Source: CAD feature listing. Evaluate the final solid. Frame: model axes, mm. A direction names the side the tool comes from. Round coordinates to 2 decimals unless told otherwise and drop trailing zeros. Loops run counter-clockwise (first coordinate to the right, second up) from the corner with the lowest first, then second, coordinate; pieces in that order, holes last. Notation, with made-up numbers: M 78.25,-39.5 L 110.25,-39.5 A22 cw 110.25,-12.5 Z; hole C 15.5,-28 d3. An arc over 180 degrees is marked long. One line per item, written item: value.
from build123d import *

# Parameters (mm, degrees)
F0_R     = 2
F1_DEPTH = 25
F2_R     = 12.5
F2_R_2   = 2
F3_DEPTH = 7.5


with BuildPart() as f1:
    # F0 (on Top) → F1 (new body)
    with BuildSketch(Plane.XY):
        Circle(F0_R)
    extrude(amount=F1_DEPTH)

    # F2 (on face) → F3 (join, symmetric)
    with BuildSketch(Plane.XY.offset(25)):
        Circle(F2_R)
        Circle(F2_R_2, mode=Mode.SUBTRACT)
    extrude(amount=F3_DEPTH, both=True)


solid = f1.part
1. Pull-direction query (Y, two-part tool) for faces 3 (the face through (0, -3, 17.5)), 4 (the face through (0, -2, 9)), 5 (the face through (0, 0, 25)); classes: released by +Y, released by -Y, zero draft, split by the parting line, or undercut.
Report:
face 3: zero draft
face 4: split by the parting line
face 5: undercut
2. Ray query, line 1 (Y direction, x = 0, z = 27); line 2 (Z direction, x = 7.5, y = -0.25); line 3 (Z direction, x = 0.75, y = -1.25). Return the intervals inside material, ascending. Write a range as [from, to].
Report:
line 1: y = [-12.5, -2], [2, 12.5]
line 2: z = [17.5, 32.5]
line 3: z = [0, 25]
3. Section query C-C (z = 18.5). Return the cut outline in (x, y), and give its area (3 significant figures).
Report:
outline: C 0,0 d25
area: 491 mm2
4. Reachability of faces 1 (the face through (0, -2, 29)), 2 (the face through (0, -3, 32.5)) from +Z, -Z, +X, -X, +Y, -Y: full face, straight path, thin tool, end or side. Return the list, or none.
Report:
face 1: +Z
face 2: +Z, +X, -X, +Y, -Y
5. Section query A-A (x = 0). Return the cut outline in (y, z), and give its area (3 significant figures).
Report:
outline: M -12.5,17.5 L -2,17.5 L -2,0 L 2,0 L 2,17.5 L 12.5,17.5 L 12.5,32.5 L 2,32.5 L 2,25 L -2,25 L -2,32.5 L -12.5,32.5 Z
area: 415 mm2
6. Pin query (flat end, axial travel): pin 1 (5 mm diameter, centred on x = -4.5, y = 6.5, fed in from -Z); pin 2 (10 mm diameter, centred on y = -7.5, z = 16.5, fed in from -X); pin 3 (3 mm diameter, centred on x = 8.5, z = 21, fed in from +Y). Return the tip coordinate at first contact, or that it passes through.
Report:
pin 1: stops at z = 17.5
pin 2: stops at x = -12.23
pin 3: stops at y = 10.36
7. Section query D-D (z = 5.5). Return the cut outline in (x, y).
Report:
outline: C 0,0 d4
